Check sheet for the modelled part. Datum: model origin and axes. Units: mm. A direction names the side the tool comes from. Give positions to 0.01 mm unless a question says otherwise; leave off trailing zeros. Loops run counter-clockwise (first coordinate to the right, second up) from the corner with the lowest first, then second, coordinate; pieces in that order, holes last. Notation, with made-up numbers: M 67.25,60 L 105.25,60 A16 cw 105.25,70 Z; hole C 2.25,-8.5 d9. An arc over 180 degrees is marked long. Put each result on its own line as item: value. Start each with the question number.
```python
from build123d import *

# Parameters (mm, degrees)
F0_R     = 3.25
F1_DEPTH = 1
F2_DEPTH = 8.5
F3_DEPTH = 3.8
F4_R     = 1.25
F5_DEPTH = 9.8


with BuildPart() as f1:
    # F0 (on Top) → F1 (new body)
    with BuildSketch(Plane.XY):
        with BuildLine():
            ThreePointArc((-3.9, 10.5523694022), (0, 11.25), (3.9, 10.5523694022))
            Line((3.9, 10.5523694022), (3.9, 11.6126009145))
            ThreePointArc((3.9, 11.6126009145), (0, 12.25), (-3.9, 11.6126009145))
            Line((-3.9, 11.6126009145), (-3.9, 10.5523694022))
        make_face()
        with BuildLine():
            ThreePointArc((-3.9, 11.6126009145), (0, 12.25), (3.9, 11.6126009145))
            Line((3.9, 11.6126009145), (3.9, 13.25))
            Line((3.9, 13.25), (-3.9, 13.25))
            Line((-3.9, 13.25), (-3.9, 11.6126009145))
        make_face()
        with BuildLine():
            ThreePointArc((-5.0059832106, 10.0748514677), (-4.4593878595, 10.3284248518), (-3.9, 10.5523694022))
            Line((-3.9, 10.5523694022), (-3.9, 11.6126009145))
            ThreePointArc((-3.9, 11.6126009145), (-4.4042152746, 11.4308961947), (-4.9, 11.2273104526))
            ThreePointArc((-4.9, 11.2273104526), (-5.3725531584, 11.0090041584), (-5.835405231, 10.7708191791))
            Line((-5.835405231, 10.7708191791), (-5.0059832106, 10.0748514677))
        make_face()
        with BuildLine():
            Line((3.9, 13.25), (3.9, 11.6126009145))
            ThreePointArc((3.9, 11.6126009145), (4.4042152746, 11.4308961947), (4.9, 11.2273104526))
            Line((4.9, 11.2273104526), (4.9, 19.25))
            Line((4.9, 19.25), (-4.9, 19.25))
            Line((-4.9, 19.25), (-4.9, 11.2273104526))
            ThreePointArc((-4.9, 11.2273104526), (-4.4042152746, 11.4308961947), (-3.9, 11.6126009145))
            Line((-3.9, 11.6126009145), (-3.9, 13.25))
            Line((-3.9, 13.25), (3.9, 13.25))
        make_face()
        with BuildLine():
            ThreePointArc((4.9, 10.1268208239), (9.5311987704, 5.9765165439), (11.25, 0))
            ThreePointArc((11.25, 0), (0, -11.25), (-11.25, 0))
            ThreePointArc((-11.25, 0), (-11.1346768386, 1.6066958954), (-10.7910716977, 3.1804514796))
            Line((-10.7910716977, 3.1804514796), (-11.6204937182, 3.8764191911))
            ThreePointArc((-11.6204937182, 3.8764191911), (-1.9636002587, -12.0915993162), (12.25, 0))
            ThreePointArc((12.25, 0), (10.249085325, 6.7096013294), (4.9, 11.2273104526))
            ThreePointArc((4.9, 11.2273104526), (4.4042152746, 11.4308961947), (3.9, 11.6126009145))
            Line((3.9, 11.6126009145), (3.9, 10.5523694022))
            ThreePointArc((3.9, 10.5523694022), (4.4051416434, 10.3516775018), (4.9, 10.1268208239))
        make_face()
        with BuildLine():
            Line((-11.6204937182, 3.8764191911), (-10.7910716977, 3.1804514796))
            ThreePointArc((-10.7910716977, 3.1804514796), (-8.6179999851, 7.231360609), (-5.0059832106, 10.0748514677))
            Line((-5.0059832106, 10.0748514677), (-5.835405231, 10.7708191791))
            ThreePointArc((-5.835405231, 10.7708191791), (-9.3840444282, 7.8741482187), (-11.6204937182, 3.8764191911))
        make_face()
        with BuildLine():
            ThreePointArc((10.25, 0), (8.8115690998, 5.2362916267), (4.9, 9.0029161942))
            ThreePointArc((4.9, 9.0029161942), (-5.2362916267, 8.8115690998), (-10.25, 0))
            ThreePointArc((-10.25, 0), (0, -10.25), (10.25, 0))
        make_face()
        Circle(F0_R, mode=Mode.SUBTRACT)
        with BuildLine():
            Line((4.9, 9.0029161942), (4.9, 10.1268208239))
            ThreePointArc((4.9, 10.1268208239), (4.4051416434, 10.3516775018), (3.9, 10.5523694022))
            ThreePointArc((3.9, 10.5523694022), (0, 11.25), (-3.9, 10.5523694022))
            ThreePointArc((-3.9, 10.5523694022), (-4.4593878595, 10.3284248518), (-5.0059832106, 10.0748514677))
            ThreePointArc((-5.0059832106, 10.0748514677), (-8.6179999851, 7.231360609), (-10.7910716977, 3.1804514796))
            ThreePointArc((-10.7910716977, 3.1804514796), (-11.1346768386, 1.6066958954), (-11.25, 0))
            Line((-11.25, 0), (-10.25, 0))
            ThreePointArc((-10.25, 0), (-5.2362916267, 8.8115690998), (4.9, 9.0029161942))
        make_face()
        with BuildLine():
            ThreePointArc((-11.25, 0), (0, -11.25), (11.25, 0))
            ThreePointArc((11.25, 0), (9.5311987704, 5.9765165439), (4.9, 10.1268208239))
            Line((4.9, 10.1268208239), (4.9, 9.0029161942))
            ThreePointArc((4.9, 9.0029161942), (8.8115690998, 5.2362916267), (10.25, 0))
            ThreePointArc((10.25, 0), (0, -10.25), (-10.25, 0))
            Line((-10.25, 0), (-11.25, 0))
        make_face()
    extrude(amount=-F1_DEPTH)

    # F0 (on Top) → F2 (join)
    with BuildSketch(Plane.XY):
        with BuildLine():
            ThreePointArc((-5.0059832106, 10.0748514677), (-4.4593878595, 10.3284248518), (-3.9, 10.5523694022))
            Line((-3.9, 10.5523694022), (-3.9, 11.6126009145))
            ThreePointArc((-3.9, 11.6126009145), (-4.4042152746, 11.4308961947), (-4.9, 11.2273104526))
            ThreePointArc((-4.9, 11.2273104526), (-5.3725531584, 11.0090041584), (-5.835405231, 10.7708191791))
            Line((-5.835405231, 10.7708191791), (-5.0059832106, 10.0748514677))
        make_face()
        with BuildLine():
            Line((3.9, 13.25), (3.9, 11.6126009145))
            ThreePointArc((3.9, 11.6126009145), (4.4042152746, 11.4308961947), (4.9, 11.2273104526))
            Line((4.9, 11.2273104526), (4.9, 19.25))
            Line((4.9, 19.25), (-4.9, 19.25))
            Line((-4.9, 19.25), (-4.9, 11.2273104526))
            ThreePointArc((-4.9, 11.2273104526), (-4.4042152746, 11.4308961947), (-3.9, 11.6126009145))
            Line((-3.9, 11.6126009145), (-3.9, 13.25))
            Line((-3.9, 13.25), (3.9, 13.25))
        make_face()
        with BuildLine():
            ThreePointArc((4.9, 10.1268208239), (9.5311987704, 5.9765165439), (11.25, 0))
            ThreePointArc((11.25, 0), (0, -11.25), (-11.25, 0))
            ThreePointArc((-11.25, 0), (-11.1346768386, 1.6066958954), (-10.7910716977, 3.1804514796))
            Line((-10.7910716977, 3.1804514796), (-11.6204937182, 3.8764191911))
            ThreePointArc((-11.6204937182, 3.8764191911), (-1.9636002587, -12.0915993162), (12.25, 0))
            ThreePointArc((12.25, 0), (10.249085325, 6.7096013294), (4.9, 11.2273104526))
            ThreePointArc((4.9, 11.2273104526), (4.4042152746, 11.4308961947), (3.9, 11.6126009145))
            Line((3.9, 11.6126009145), (3.9, 10.5523694022))
            ThreePointArc((3.9, 10.5523694022), (4.4051416434, 10.3516775018), (4.9, 10.1268208239))
        make_face()
    extrude(amount=F2_DEPTH)

    # F0 (on Top) → F3 (join)
    with BuildSketch(Plane.XY):
        with BuildLine():
            ThreePointArc((-11.25, 0), (0, -11.25), (11.25, 0))
            ThreePointArc((11.25, 0), (9.5311987704, 5.9765165439), (4.9, 10.1268208239))
            Line((4.9, 10.1268208239), (4.9, 9.0029161942))
            ThreePointArc((4.9, 9.0029161942), (8.8115690998, 5.2362916267), (10.25, 0))
            ThreePointArc((10.25, 0), (0, -10.25), (-10.25, 0))
            Line((-10.25, 0), (-11.25, 0))
        make_face()
    extrude(amount=F3_DEPTH)

    # F4 (on face) → F5 (cut, through all)
    with BuildSketch(Plane.YZ.offset(4.9)):
        with BuildLine():
            ThreePointArc((14.75, 8.5), (17.9463721422, 7.0215630821), (19.25, 3.75))
            Line((19.25, 3.75), (19.25, 8.5))
            Line((19.25, 8.5), (14.75, 8.5))
        make_face()
        with BuildLine():
            ThreePointArc((19.25, 3.75), (17.9463721422, 0.4784369179), (14.75, -1))
            Line((14.75, -1), (19.25, -1))
            Line((19.25, -1), (19.25, 3.75))
        make_face()
        with Locations((17, 3.75)):
            Circle(F4_R)
    extrude(amount=-F5_DEPTH, mode=Mode.SUBTRACT)


solid = f1.part
```
Q1. Thickness scan on line 1 along Y through (x, z) = (0.5, 2.75); line 2 along Y through (x, z) = (-3.5, 3); line 3 along Z through (x, y) = (3.25, 13). Record the ranges inside material, lowest first. Write a range as [from, to].
Q2. Access from +Z, -Z, +X, -X, +Y, -Y to the whole of each face (thin tool, end or side, straight path). Record for faces 1 (the face through (-5.43, 10.43, 4.19)), 2 (the face through (4.9, 14, 4)), 3 (the face through (0, 13.25, 4)).
Q3. Section check C-C, the plane x = 2.5. Record the cut outline in (y, z).
Q4. Section check A-A, the plane x = 0. Record the cut outline in (y, z).
Q5. Section check B-B, the plane y = 17. Record the cut outline in (x, z).
Q6. Section check D-D, the plane z = 6.5. Record the cut outline in (x, y).
Q7. Mould release check, pull along Y, two halves, no side actions. Record for faces 4 (the face through (-4.9, 14, 4)), 5 (the face through (-11, 0, 2)), 6 (the face through (-11.2, 3.524, 4.19)), 7 (the face through (3.9, 12, 4)): pulls with the +Y half, pulls with the -Y half, needs draft (parallel to the pull), parting line crosses it, or undercut.
Q8. Depth check by flat-ended pin: P1, Ø4, axis at x = -3.5, y = -8, coming from the +Z side; P2, Ø2, axis at y = 11.5, z = 3.5, coming from the +X side; P3, Ø7.5, axis at x = 0, y = 0, coming from the +Z side; P4, Ø4, axis at x = 0.5, z = 5.5, coming from the -Y side. Enter the tip coordinate at first touch or a pass-through.
Found:
1. line 1: y = [-12.24, -10.24], [13.25, 16.25], [17.75, 19.14]
1. line 2: y = [-11.74, -9.63], [13.25, 16], [18, 19.19]
1. line 3: z = [-1, 0]
2. face 1: +Z, -X
2. face 2: +Z, -Z, +X, +Y
2. face 3: +Z
3. outline: M -11.99,-1 L -2.08,-1 L -2.08,0 L -9.94,0 L -9.94,3.8 L -10.97,3.8 L -10.97,8.5 L -11.99,8.5 Z; M 2.08,-1 L 14.75,-1 A4.76 ccw 14.75,8.5 L 13.25,8.5 L 13.25,0 L 2.08,0 Z; hole C 17,3.75 d2.5
4. outline: M -12.25,-1 L -3.25,-1 L -3.25,0 L -10.25,0 L -10.25,3.8 L -11.25,3.8 L -11.25,8.5 L -12.25,8.5 Z; M 3.25,-1 L 14.75,-1 A4.76 ccw 14.75,8.5 L 13.25,8.5 L 13.25,0 L 3.25,0 Z; hole C 17,3.75 d2.5
5. outline: M -4.9,-0.29 L 4.9,-0.29 L 4.9,2.5 L -4.9,2.5 Z; M -4.9,5 L 4.9,5 L 4.9,7.79 L -4.9,7.79 Z
6. outline: M -11.62,3.88 A12.25 ccw long 4.9,11.23 L 4.9,18.37 L -4.9,18.37 L -4.9,11.23 A12.25 ccw -5.84,10.77 L -5.01,10.07 A11.25 cw -3.9,10.55 L -3.9,13.25 L 3.9,13.25 L 3.9,10.55 A11.25 cw long -10.79,3.18 Z
7. face 4: needs draft
7. face 5: undercut
7. face 6: pulls with the +Y half
7. face 7: undercut
8. P1: stops at z = 3.8
8. P2: stops at x = 6.31
8. P3: stops at z = 0
8. P4: stops at y = -12.25
